from build123d import *

# Parameters (mm, degrees)
SKETCH1_W           = 202
SKETCH1_H           = 102
BOSS_EXTRUDE1_DEPTH = 2
SKETCH2_W           = 15
SKETCH2_H           = 1
SKETCH2_W_2         = 1
SKETCH2_H_2         = 15
BOSS_EXTRUDE2_DEPTH = 11.6
SKETCH3_W           = 202
SKETCH3_H           = 2
BOSS_EXTRUDE3_DEPTH = 10
SKETCH10_W          = 10
SKETCH10_H          = 2
CUT_EXTRUDE1_DEPTH  = 8
SKETCH12_R          = 1.75
BOSS_EXTRUDE5_DEPTH = 2
SKETCH13_W          = 15
SKETCH13_H          = 10
CUT_EXTRUDE2_DEPTH  = 119.560364372


with BuildPart() as part:
    # Sketch1 → Boss-Extrude1 (new body)
    with BuildSketch(Plane(origin=(0, 0, 0), x_dir=(1, 0, 0), z_dir=(0, 1, 0))):
        Rectangle(SKETCH1_W, SKETCH1_H)
    extrude(amount=BOSS_EXTRUDE1_DEPTH)

    # Sketch2 → Boss-Extrude2 (add)
    with BuildSketch(Plane(origin=(0, 2, 0), x_dir=(1, 0, 0), z_dir=(0, 1, 0))):
        with Locations((-67.5, 50.5)):
            Rectangle(SKETCH2_W, SKETCH2_H)
        with Locations((-67.5, -50.5)):
            Rectangle(SKETCH2_W, SKETCH2_H)
        with Locations((67.5, -50.5)):
            Rectangle(SKETCH2_W, SKETCH2_H)
        with Locations((67.5, 50.5)):
            Rectangle(SKETCH2_W, SKETCH2_H)
        with Locations((100.5, 0)):
            Rectangle(SKETCH2_W_2, SKETCH2_H_2)
        with Locations((-100.5, 0)):
            Rectangle(SKETCH2_W_2, SKETCH2_H_2)
    extrude(amount=BOSS_EXTRUDE2_DEPTH)

    # Sketch3 → Boss-Extrude3 (add)
    with BuildSketch(Plane.XY.offset(51)):
        with Locations((0, 1)):
            Rectangle(SKETCH3_W, SKETCH3_H)
    extrude(amount=BOSS_EXTRUDE3_DEPTH)

    # Sketch10 → Cut-Extrude1 (cut)
    with BuildSketch(Plane.ZY.offset(101)):
        with Locations((56, 1)):
            Rectangle(SKETCH10_W, SKETCH10_H)
    cut_extrude1 = extrude(amount=-CUT_EXTRUDE1_DEPTH, mode=Mode.SUBTRACT)

    # Mirror3: Cut-Extrude1 across plane
    add(cut_extrude1.mirror(Plane.ZY), mode=Mode.SUBTRACT)

    # Sketch12 → Boss-Extrude5 (add)
    with BuildSketch(Plane.ZY.offset(93)):
        with BuildLine():
            Line((61, 2), (61, 7))
            ThreePointArc((61, 7), (57, 11), (53, 7))
            Line((53, 7), (53, 2))
            Line((53, 2), (61, 2))
        make_face()
        with Locations((57, 7)):
            Circle(SKETCH12_R, mode=Mode.SUBTRACT)
    boss_extrude5 = extrude(amount=-BOSS_EXTRUDE5_DEPTH)

    # Mirror4: Boss-Extrude5 across plane
    add(boss_extrude5.mirror(Plane.ZY))

    # Sketch13 → Cut-Extrude2 (cut, through all)
    with BuildSketch(Plane(origin=(0, 2, 0), x_dir=(1, 0, 0), z_dir=(0, 1, 0))):
        with Locations((-67.5, -56)):
            Rectangle(SKETCH13_W, SKETCH13_H)
        with Locations((67.5, -56)):
            Rectangle(SKETCH13_W, SKETCH13_H)
    extrude(amount=-CUT_EXTRUDE2_DEPTH, mode=Mode.SUBTRACT)


solid = part.part
Geometry check sheet. Reference: the model listing, model coordinates, mm. A direction names the side the tool comes from. Coordinates: 2 decimals unless noted, no trailing zeros. Order: outer loops, then holes, each group sorted by start corner. A loop starts at its lowest first (then second) coordinate and runs counter-clockwise, first axis right, second up. Notation, with made-up numbers: (-5.75, 58) -> (16.25, 58) arc R12 cw to (16.25, 65) -> close; hole circle Ø8 at (-16.5, 86.5). An arc over 180 degrees is marked (long way). Use a Markdown table: item, result. Add a question column.
1. Material ranges on L1, parallel to Y at x = -91.75, z = 57; L2, parallel to X at y = 3.5, z = -1; L3, parallel to Y at x = 1, z = -2, recorded low to high.
2. Cross-section at C-C (x = 25.5). Enter the section's corners in (y, z), and give its area (3 significant figures).
3. Cross-section at B-B (z = 0.5). Enter the section's corners in (x, y).
4. Cross-section at D-D (z = -32). Enter the section's corners in (x, y), and give its area (3 significant figures).
5. Cross-section at A-A (x = -65). Enter the section's corners in (y, z).
6. Go/stop test with flat-tipped pins: pin 1 Ø0.8 at (y, z) = (6.5, -50.5) entering from -X; pin 2 Ø2 at (x, y) = (-62.5, 9) entering from +Z; pin 3 Ø0.5 at (y, z) = (5, 50.5) entering from +X. Record where each tip stops, or that it passes through.
7. Set-up check for faces 1 (the face through (-93, 4, 57)), 2 (the face through (91, 5, 57)), 3 (the face through (93, 4, 57)), 4 (the face through (-86, 1, 61)), 5 (the face through (-68, 8, 50)): record each of +Z, -Z, +X, -X, +Y, -Y from which the full face is reachable in a straight line by a thin tool's end or side.
8. Mould release check, pull along Y, two halves, no side actions. Record for faces 6 (the face through (-92.014, 6.33, 58.617)), 7 (the face through (-1, 2, 4)), 8 (the face through (100, 8, 0)): pulls with the +Y half, pulls with the -Y half, needs draft (parallel to the pull), parting line crosses it, or undercut.
Filled sheet:
| question | item | result |
|---|---|---|
| 1 | L1 | 0 to 5.25, 8.75 to 11 |
| 1 | L2 | -101 to -100, 100 to 101 |
| 1 | L3 | 0 to 2 |
| 2 | outline | (0, -51) -> (2, -51) -> (2, 61) -> (0, 61) -> close |
| 2 | area | 224 mm2 |
| 3 | outline | (-101, 0) -> (101, 0) -> (101, 13.6) -> (100, 13.6) -> (100, 2) -> (-100, 2) -> (-100, 13.6) -> (-101, 13.6) -> close |
| 4 | outline | (-101, 0) -> (101, 0) -> (101, 2) -> (-101, 2) -> close |
| 4 | area | 404 mm2 |
| 5 | outline | (0, -51) -> (13.6, -51) -> (13.6, -50) -> (2, -50) -> (2, 50) -> (13.6, 50) -> (13.6, 51) -> (0, 51) -> close |
| 6 | pin 1 | x = -75 |
| 6 | pin 2 | z = 51 |
| 6 | pin 3 | x = 75 |
| 7 | face 1 | +Z, -X, +Y, -Y |
| 7 | face 2 | +Z, -Z, +Y |
| 7 | face 3 | +Z, +X, +Y, -Y |
| 7 | face 4 | +Z, +X, -X, +Y, -Y |
| 7 | face 5 | +X, -X, +Y |
| 8 | face 6 | undercut |
| 8 | face 7 | pulls with the +Y half |
| 8 | face 8 | needs draft |
